```python
from build123d import *

# Parameters (mm, degrees)
SKETCH1_W                 = 7.82
SKETCH1_H                 = 51
BOSS_EXTRUDE1_DEPTH       = 25
SKETCH2_W                 = 55
SKETCH2_H                 = 23.07
BOSS_EXTRUDE2_DEPTH       = 5
SKETCH3_W                 = 55
SKETCH3_H                 = 23.07
SKETCH3_W_2               = 51.2
SKETCH3_H_2               = 19.27
BOSS_EXTRUDE3_DEPTH       = 2
FILLET1_R                 = 10
FILLET2_R                 = 3
SKETCH4_W                 = 3
SKETCH4_H                 = 10
BOSS_EXTRUDE4_DEPTH       = 2.5
CHAMFER1_SIZE             = 1
SKETCH5_W                 = 98.213610125
SKETCH5_H                 = 151.23254193
CUT_EXTRUDE1_DEPTH        = 30
SKETCH6_W                 = 5.457780719
SKETCH6_H                 = 23.07
BOSS_EXTRUDE5_DEPTH       = 70
SKETCH7_W                 = 16.36852431
SKETCH7_H                 = 23.07
BOSS_EXTRUDE6_DEPTH       = 3
CHAMFER2_SIZE             = 13
CHAMFER2_SIZE2            = 10.908295205
CHAMFER2_OF_MIRROR1_SIZE2 = 10.908295205
CHAMFER2_OF_MIRROR1_SIZE  = 13


with BuildPart() as part:
    # Sketch1 → Boss-Extrude1 (new body)
    with BuildSketch(Plane(origin=(0, 0, 0), x_dir=(1, 0, 0), z_dir=(0, 1, 0))):
        Rectangle(SKETCH1_W, SKETCH1_H)
    extrude(amount=BOSS_EXTRUDE1_DEPTH)

    # Sketch2 → Boss-Extrude2 (add)
    with BuildSketch(Plane(origin=(0, 25, 0), x_dir=(1, 0, 0), z_dir=(0, 1, 0))):
        Rectangle(SKETCH2_W, SKETCH2_H)
    extrude(amount=BOSS_EXTRUDE2_DEPTH)

    # Sketch3 → Boss-Extrude3 (add)
    with BuildSketch(Plane(origin=(0, 30, 0), x_dir=(1, 0, 0), z_dir=(0, 1, 0))):
        Rectangle(SKETCH3_W, SKETCH3_H)
        Rectangle(SKETCH3_W_2, SKETCH3_H_2, mode=Mode.SUBTRACT)
    extrude(amount=BOSS_EXTRUDE3_DEPTH)

    # Fillet1
    fillet1_edges = [part.edges().sort_by_distance(p)[0] for p in [
        (-3.91, 25, 0),
    ]]
    fillet(fillet1_edges, radius=FILLET1_R)

    # Fillet2
    fillet2_edges = [part.edges().sort_by_distance(p)[0] for p in [
        (3.91, 25, 0),
    ]]
    fillet(fillet2_edges, radius=FILLET2_R)

    # Sketch4 → Boss-Extrude4 (add)
    with BuildSketch(Plane.ZY.offset(3.91)):
        Rectangle(SKETCH4_W, SKETCH4_H)
    extrude(amount=BOSS_EXTRUDE4_DEPTH)

    # Chamfer1
    chamfer1_edges = [part.edges().sort_by_distance(p)[0] for p in [
        (-3.91, 2.5, 1.5),
        (-3.91, 5, 0),
        (-3.91, 2.5, -1.5),
    ]]
    chamfer(chamfer1_edges, length=CHAMFER1_SIZE)

    # Sketch5 → Cut-Extrude1 (cut)
    with BuildSketch(Plane(origin=(0, -5, 0), x_dir=(-1, 0, 0), z_dir=(0, -1, 0))):
        with Locations((5.202747623, 0)):
            Rectangle(SKETCH5_W, SKETCH5_H)
    extrude(amount=-CUT_EXTRUDE1_DEPTH, mode=Mode.SUBTRACT)

    # Sketch6 → Boss-Extrude5 (add)
    with BuildSketch(Plane(origin=(0, 25, 0), x_dir=(-1, 0, 0), z_dir=(0, -1, 0))):
        with Locations((-21.087107753, 0)):
            Rectangle(SKETCH6_W, SKETCH6_H)
    boss_extrude5 = extrude(amount=BOSS_EXTRUDE5_DEPTH)

    # Sketch7 → Boss-Extrude6 (add)
    with BuildSketch(Plane(origin=(0, -45, 0), x_dir=(-1, 0, 0), z_dir=(0, -1, 0))):
        with Locations((-15.631735957, 0)):
            Rectangle(SKETCH7_W, SKETCH7_H)
    boss_extrude6 = extrude(amount=BOSS_EXTRUDE6_DEPTH)

    # Chamfer2
    chamfer2_edges = [part.edges().sort_by_distance(p)[0] for p in [
        (18.358217393, -45, 0),
    ]]
    chamfer2_side = [part.faces().sort_by_distance(p)[0] for p in [
        (18.358217393, -10, 0),
    ]]
    chamfer(chamfer2_edges, length=CHAMFER2_SIZE, length2=CHAMFER2_SIZE2, reference=chamfer2_side[0])

    # Mirror1: Boss-Extrude5, Boss-Extrude6 across plane
    add(boss_extrude5.mirror(Plane(origin=(0, 0, 0), x_dir=(0, 0, 1), z_dir=(1, 0, 0))))
    add(boss_extrude6.mirror(Plane(origin=(0, 0, 0), x_dir=(0, 0, 1), z_dir=(1, 0, 0))))

    # Chamfer2 of Mirror1
    chamfer2_of_mirror1_edges = [part.edges().sort_by_distance(p)[0] for p in [
        (-18.358217393, -45, 0),
    ]]
    chamfer(chamfer2_of_mirror1_edges, length=CHAMFER2_OF_MIRROR1_SIZE, length2=CHAMFER2_OF_MIRROR1_SIZE2)


solid = part.part
```
Input: part model. Units: mm. Frame: model coordinates. A direction names the side the tool comes from. Give positions to 0.01 mm unless a question says otherwise; leave off trailing zeros. Loops run counter-clockwise (first coordinate to the right, second up) from the corner with the lowest first, then second, coordinate; pieces in that order, holes last.
1) Section query A-A on y = -21. Return the cut outline in (x, z) (3 decimals), and give its area (3 significant figures).
A:
outline: (-23.816, -11.535) - (-18.358, -11.535) - (-18.358, 11.535) - (-23.816, 11.535) - close; (18.358, -11.535) - (23.816, -11.535) - (23.816, 11.535) - (18.358, 11.535) - close
area: 252 mm2
2) Line query: L1, parallel to X at y = 12, z = 7.75; L2, parallel to Y at x = -20, z = -7; L3, parallel to Y at x = -11, z = -3. Output: solid intervals per line, ascending.
A:
L1: x = -23.82 to -18.36, 18.36 to 23.82
L2: y = -48 to 30
L3: y = -48 to -40.77, 25 to 30
3) Section query C-C on x = -11. Return the cut outline in (y, z) (3 decimals).
A:
outline: (-48, -11.535) - (-40.769, -11.535) - (-40.769, 11.535) - (-48, 11.535) - close; (25, -11.535) - (32, -11.535) - (32, -9.635) - (30, -9.635) - (30, 9.635) - (32, 9.635) - (32, 11.535) - (25, 11.535) - close
4) Section query D-D on x = -3.5. Return the cut outline in (y, z) (3 decimals).
A:
outline: (25, -11.535) - (32, -11.535) - (32, -9.635) - (30, -9.635) - (30, 9.635) - (32, 9.635) - (32, 11.535) - (25, 11.535) - close
5) Mould query, pull axis Z, two halves, no side actions, for faces 6 (the flat face through (0, 30, 0)), 7 (the flat face through (23.816, -11, 0)), 8 (the flat face through (-20, -5, -11.535)). Classes: released by +Z, released by -Z, zero draft, split by the parting line, or undercut.
A:
face 6: undercut
face 7: zero draft
face 8: released by -Z
6) Contact query for flat-ended pins moving along their axis: pin 1 (9.5 mm diameter, centred on x = -3.5, z = 1.5, fed in from +Y); pin 2 (12 mm diameter, centred on y = -5.5, z = 3.5, fed in from +X); pin 3 (3.5 mm diameter, centred on y = -46, z = -3, fed in from -X); pin 4 (10 mm diameter, centred on x = 12, y = -13.5, fed in from +Z). Output: stop coordinate, or through.
A:
pin 1: stops at y = 30
pin 2: stops at x = 23.82
pin 3: stops at x = -23.82
pin 4: passes through
7) Reachability of faces 1 (the flat face through (26, 25, 0)), 2 (the flat face through (0, 25, 0)), 3 (the flat face through (-7.447, -46, 0)), 4 (the flat face through (0, 31, 9.635)), 5 (the flat face through (-26, 25, 0)) from +Z, -Z, +X, -X, +Y, -Y: full face, straight path, thin tool, end or side. Return the list, or none.
A:
face 1: +Z, -Z, +X, -Y
face 2: +Z, -Z
face 3: +Z, -Z, -Y
face 4: +Y
face 5: +Z, -Z, -X, -Y
